Check sheet for the modelled part. Datum: model origin and axes. Units: mm. Round coordinates to 2 decimals unless told otherwise and drop trailing zeros. Write each loop counter-clockwise with the first axis right and the second up, starting at its lowest first coordinate (ties: lowest second). Pieces come first, ordered by that corner, then holes. Notation, with made-up numbers: M -22.5,83.25 L -17.5,83.25 A29 ccw -17.5,120.25 Z; hole C 81.5,14 d10. An arc over 180 degrees is marked long. Answer in a Markdown table with one row per item.
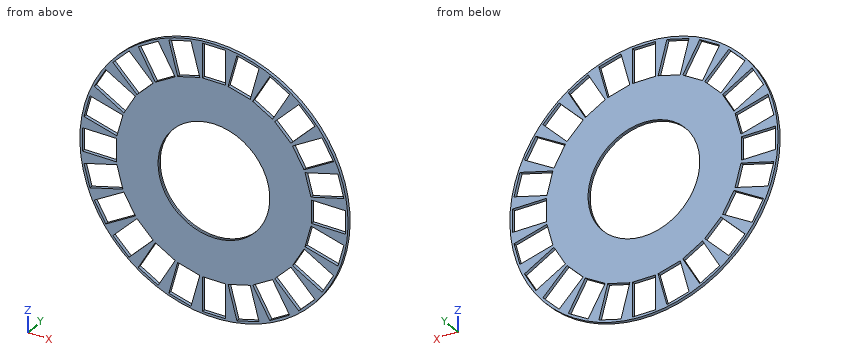
```python
from build123d import *

# Parameters (mm, degrees)
SKETCH1_R           = 120
BOSS_EXTRUDE1_DEPTH = 1.5
SKETCH6_W           = 30.5
SKETCH6_H           = 20.5
SKETCH6_W_2         = 20.5
SKETCH6_H_2         = 30.5
CUT_EXTRUDE1_DEPTH  = 10.5


with BuildPart() as part:
    # Sketch1 → Boss-Extrude1 (new, symmetric)
    with BuildSketch(Plane(origin=(0, 0, 0), x_dir=(1, 0, 0), z_dir=(0, 1, 0))):
        with Locations(Location((98.638798209, 0, 0), (0, 0, 270))):
            Circle(SKETCH1_R)
        with BuildLine():
            ThreePointArc((118.472374081, -45.898031201), (49.529315887, -9.394612605), (100.131404816, 49.97771629))
            ThreePointArc((100.131404816, 49.97771629), (147.748280532, 9.394612605), (118.472374081, -45.898031201))
        make_face(mode=Mode.SUBTRACT)
    extrude(amount=BOSS_EXTRUDE1_DEPTH, both=True)

    # Sketch6 → Cut-Extrude1 (cut)
    with BuildSketch(Plane(origin=(0, 1.5, 0), x_dir=(1, 0, 0), z_dir=(0, 1, 0))):
        with Locations((-3.75, 0)):
            Rectangle(SKETCH6_W, SKETCH6_H)
        Polygon((-12.338659942, 40.347901139), (-17.644450367, 20.5464217), (11.816287335, 12.652440824), (17.122077759, 32.453920263), align=None)
        Polygon((1.885610489, 67.696159493), (-8.364389511, 49.942638716), (18.049385305, 34.692638716), (28.299385305, 52.446159493), align=None)
        Polygon((22.703450772, 90.431036452), (8.207761758, 75.935347437), (29.774518584, 54.368590611), (44.270207598, 68.864279625), align=None)
        Polygon((48.696159493, 107.00318772), (30.942638716, 96.75318772), (46.192638716, 70.339412904), (63.946159493, 80.589412904), align=None)
        Polygon((78.092376509, 116.283248576), (58.29089707, 110.977458152), (66.184877946, 81.51672045), (85.986357385, 86.822510874), align=None)
        with Locations((98.638798209, 102.388798209)):
            Rectangle(SKETCH6_W_2, SKETCH6_H_2)
        Polygon((138.986699348, 110.977458152), (119.185219909, 116.283248576), (111.291239034, 86.822510874), (131.092718473, 81.51672045), align=None)
        Polygon((166.334957703, 96.75318772), (148.581436925, 107.00318772), (133.331436925, 80.589412904), (151.084957703, 70.339412904), align=None)
        Polygon((189.069834661, 75.935347437), (174.574145646, 90.431036452), (153.00738882, 68.864279625), (167.503077834, 54.368590611), align=None)
        Polygon((205.641985929, 49.942638716), (195.391985929, 67.696159493), (168.978211114, 52.446159493), (179.228211114, 34.692638716), align=None)
        Polygon((214.922046785, 20.5464217), (209.616256361, 40.347901139), (180.155518659, 32.453920263), (185.461309084, 12.652440824), align=None)
        with Locations((201.027596418, 0)):
            Rectangle(SKETCH6_W, SKETCH6_H)
        Polygon((209.616256361, -40.347901139), (214.922046785, -20.5464217), (185.461309084, -12.652440824), (180.155518659, -32.453920263), align=None)
        Polygon((195.391985929, -67.696159493), (205.641985929, -49.942638716), (179.228211114, -34.692638716), (168.978211114, -52.446159493), align=None)
        Polygon((174.574145646, -90.431036451), (189.069834661, -75.935347437), (167.503077835, -54.368590611), (153.00738882, -68.864279625), align=None)
        Polygon((148.581436925, -107.00318772), (166.334957703, -96.75318772), (151.084957703, -70.339412904), (133.331436925, -80.589412904), align=None)
        Polygon((119.185219909, -116.283248576), (138.986699348, -110.977458152), (131.092718473, -81.51672045), (111.291239034, -86.822510874), align=None)
        with Locations((98.638798209, -102.388798209)):
            Rectangle(SKETCH6_W_2, SKETCH6_H_2)
        Polygon((58.29089707, -110.977458152), (78.092376509, -116.283248576), (85.986357385, -86.822510874), (66.184877946, -81.51672045), align=None)
        Polygon((30.942638716, -96.75318772), (48.696159493, -107.00318772), (63.946159493, -80.589412904), (46.192638716, -70.339412904), align=None)
        Polygon((8.207761758, -75.935347437), (22.703450772, -90.431036452), (44.270207598, -68.864279625), (29.774518584, -54.368590611), align=None)
        Polygon((-8.364389511, -49.942638716), (1.885610489, -67.696159493), (28.299385305, -52.446159493), (18.049385305, -34.692638716), align=None)
        Polygon((-17.644450367, -20.5464217), (-12.338659942, -40.347901139), (17.122077759, -32.453920263), (11.816287335, -12.652440824), align=None)
    extrude(amount=-CUT_EXTRUDE1_DEPTH, mode=Mode.SUBTRACT)


solid = part.part
```
1. Section check B-B, the plane x = 201.5. Record the cut outline in (y, z), and give its area (3 significant figures).
Found:
| item | result |
|---|---|
| outline | M -1.5,-61.8 L 1.5,-61.8 L 1.5,-57.12 L -1.5,-57.12 Z; M -1.5,-47.55 L 1.5,-47.55 L 1.5,-38.17 L -1.5,-38.17 Z; M -1.5,-16.95 L 1.5,-16.95 L 1.5,-10.25 L -1.5,-10.25 Z; M -1.5,10.25 L 1.5,10.25 L 1.5,16.95 L -1.5,16.95 Z; M -1.5,38.17 L 1.5,38.17 L 1.5,47.55 L -1.5,47.55 Z; M -1.5,57.12 L 1.5,57.12 L 1.5,61.8 L -1.5,61.8 Z |
| area | 125 mm2 |
2. Go/stop test with flat-tipped pins: pin 1 (0.9 mm diameter, centred on y = 0, z = 96.5, fed in from +X); pin 2 (0.9 mm diameter, centred on x = 208, y = 0.5, fed in from +Z); pin 3 (0.9 mm diameter, centred on y = 0, z = -3.5, fed in from -X). Record where each tip stops, or that it passes through.
Found:
| item | result |
|---|---|
| pin 1 | stops at x = 170.57 |
| pin 2 | stops at z = 50.38 |
| pin 3 | stops at x = -21.32 |
3. Section check D-D, the plane y = -0.75. Count the separate pieces of the cut face and the enclosed holes in it, and give its area (3 significant figures).
Found:
| item | result |
|---|---|
| separate pieces | 1 |
| enclosed holes | 25 |
| area | 22,400 mm2 |
4. Section check A-A, the plane z = 0. Record the cut outline in (x, y), and give its area (3 significant figures).
Found:
| item | result |
|---|---|
| outline | M -21.36,-1.5 L -19,-1.5 L -19,1.5 L -21.36,1.5 Z; M 11.5,-1.5 L 48.64,-1.5 L 48.64,1.5 L 11.5,1.5 Z; M 148.64,-1.5 L 185.78,-1.5 L 185.78,1.5 L 148.64,1.5 Z; M 216.28,-1.5 L 218.64,-1.5 L 218.64,1.5 L 216.28,1.5 Z |
| area | 237 mm2 |
5. Section check C-C, the plane x = 144.5. Record the cut outline in (y, z), and give its area (3 significant figures).
Found:
| item | result |
|---|---|
| outline | M -1.5,-110.89 L 1.5,-110.89 L 1.5,-99.93 L -1.5,-99.93 Z; M -1.5,-74.14 L 1.5,-74.14 L 1.5,-19.92 L -1.5,-19.92 Z; M -1.5,19.92 L 1.5,19.92 L 1.5,74.14 L -1.5,74.14 Z; M -1.5,99.93 L 1.5,99.93 L 1.5,110.89 L -1.5,110.89 Z |
| area | 391 mm2 |
6. Scan lines: L1, parallel to X at y = -0.4, z = 0; L2, parallel to Z at x = 120.5, y = -0.7; L3, parallel to X at y = 0.5, z = -53.5. Record each from-to range of solid material in increasing order.
Found:
| item | result |
|---|---|
| L1 | x = -21.36 to -19, 11.5 to 48.64, 148.64 to 185.78, 216.28 to 218.64 |
| L2 | z = -117.99 to -115.93, -84.36 to -44.97, 44.97 to 84.36, 115.93 to 117.99 |
| L3 | x = -8.78 to -6.31, 26.47 to 170.8, 203.59 to 206.05 |
